```python
from build123d import *

# Parameters (mm, degrees)
BOSS_EXTRU_1_DEPTH      = 100
ESQUISSE3_R             = 2
ENL_V_MAT_EXTRU_2_DEPTH = 115.052675119
ESQUISSE7_W             = 5.5
ESQUISSE7_H             = 20.980762114
BOSS_EXTRU_3_DEPTH      = 29.226497
BOSS_EXTRU_4_OUTLINE_W  = 5.5
BOSS_EXTRU_4_OUTLINE_H  = 18.169872981
BOSS_EXTRU_4_DEPTH      = 10.490381057
CONG_2_R                = 40
CONG_3_R                = 40
CONG_4_R                = 5
CONG_5_RADIUS           = 5
CONG_5_LENGTH           = 100
ESQUISSE9_R             = 1.5
ENL_V_MAT_EXTRU_3_DEPTH = 112.741489915
CONG_6_R                = 1
CONG_7_R                = 1
CONG_8_R                = 30


# Read off the part's stored shape, not the designer's step: Boss.-Extru.4
with BuildPart() as part:
    # Esquisse1 → Boss.-Extru.1 (new body)
    with BuildSketch(Plane.XY):
        with BuildLine():
            Line((0, 0), (0, -24.226497308))
            ThreePointArc((0, -24.226497308), (1.339745962, -29.226497308), (5, -32.886751346))
            Line((5, -32.886751346), (30.310889132, -47.5))
            Line((30.310889132, -47.5), (35.310889132, -38.839745962))
            Line((35.310889132, -38.839745962), (10, -24.226497308))
            Line((10, -24.226497308), (10, 0))
            Line((10, 0), (0, 0))
        make_face()
    extrude(amount=BOSS_EXTRU_1_DEPTH)

    # Esquisse3 → Enlèv. mat.-Extru.2 (cut, through all)
    with BuildSketch(Plane(origin=(-7.990381057, -13.839745962, 0), x_dir=(0.86602540378444, -0.4999999999999978, 0), z_dir=(0.4999999999999978, 0.86602540378444, 0))):
        with Locations(Location((35.386751346, -50, 0), (0, 0, 180))):
            Circle(ESQUISSE3_R)
    extrude(amount=-ENL_V_MAT_EXTRU_2_DEPTH, mode=Mode.SUBTRACT)

    # Esquisse7 → Boss.-Extru.3 (add)
    with BuildSketch(Plane(origin=(43.301270189, -25, 0), x_dir=(0, 0, -1), z_dir=(0.86602540378444, -0.49999999999999756, 0))):
        with Locations((-97.25, -5.490381057)):
            Rectangle(ESQUISSE7_W, ESQUISSE7_H)
        with Locations((-2.75, -5.490381057)):
            Rectangle(ESQUISSE7_W, ESQUISSE7_H)
    extrude(amount=-BOSS_EXTRU_3_DEPTH)

    # Boss.-Extru.4 outline → Boss.-Extru.4 (add)
    with BuildSketch(Plane(origin=(10, 0, 0), x_dir=(0, 0, -1), z_dir=(1, 0, 0))):
        with Locations((-2.75, -15.141560818)):
            Rectangle(BOSS_EXTRU_4_OUTLINE_W, BOSS_EXTRU_4_OUTLINE_H)
        with Locations((-97.25, -15.141560818)):
            Rectangle(BOSS_EXTRU_4_OUTLINE_W, BOSS_EXTRU_4_OUTLINE_H)
    extrude(amount=BOSS_EXTRU_4_DEPTH)

    # Congé2
    # the kernel refuses this fillet: 40 mm, written as the material it takes off along each edge
    with BuildSketch(Plane(origin=(20.490381057, -6.056624327, 32.29491991), x_dir=(-1, 0, 0), z_dir=(0, 0, -1))) as cong_2_piece_1_section:
        with BuildLine():
            CenterArc((CONG_2_R * 0.267949192431, -CONG_2_R), CONG_2_R, 90, 30)
            Line((-CONG_2_R * 0.232050807569, -CONG_2_R * 0.133974596216), (0, 0))
            Line((0, 0), (CONG_2_R * 0.267949192431, 0))
        make_face()
    cong_2_piece_1 = extrude(amount=59.089839821, mode=Mode.PRIVATE)
    cong_2_piece_1 = split(cong_2_piece_1, bisect_by=Plane(origin=(10, -7.066001807, 2.75), z_dir=(1, 0, 0)), keep=Keep.TOP, mode=Mode.PRIVATE)
    add(cong_2_piece_1, mode=Mode.SUBTRACT)
    with BuildSketch(Plane(origin=(20.490381057, -6.056624327, 67.70508009), x_dir=(-1, 0, 0), z_dir=(0, 0, 1))) as cong_2_piece_2_section:
        with BuildLine():
            CenterArc((CONG_2_R * 0.267949192431, CONG_2_R), CONG_2_R, 240, 30)
            Line((-CONG_2_R * 0.232050807569, CONG_2_R * 0.133974596216), (0, 0))
            Line((0, 0), (CONG_2_R * 0.267949192431, 0))
        make_face()
    cong_2_piece_2 = extrude(amount=59.089839821, mode=Mode.PRIVATE)
    cong_2_piece_2 = split(cong_2_piece_2, bisect_by=Plane(origin=(10, -7.066001807, 97.25), z_dir=(1, 0, 0)), keep=Keep.TOP, mode=Mode.PRIVATE)
    add(cong_2_piece_2, mode=Mode.SUBTRACT)

    # Congé3
    # the kernel refuses this fillet: 40 mm, written as the material it takes off along each edge
    with BuildSketch(Plane(origin=(45.801270189, -20.669872981, -2.92475776), x_dir=(-0.8660254037844402, 0.49999999999999756, 0), z_dir=(0, 0, 1))) as cong_3_piece_1:
        with BuildLine():
            CenterArc((38.969903104, 40), CONG_3_R, 193.031161189, 76.968838811)
            Line((0, 30.980762114), (-0.779398062, 30.800377356))
            ThreePointArc((-0.779398062, 30.800377356), (-0.8, 15.490381057), (-0.8, 0))
            Line((-0.8, 0), (0, -0.8))
            Line((0, -0.8), (38.969903104, -0.8))
            Line((38.969903104, -0.8), (38.969903104, 0))
        make_face()
    extrude(amount=200.349515521, mode=Mode.SUBTRACT)

    # Congé4
    cong_4_edges = [part.edges().sort_by_distance(p)[0] for p in [
        (30.310889132, -47.5, 50),
    ]]
    fillet(cong_4_edges, radius=CONG_4_R)

    # Congé5: full round fillet: the end face becomes a half cylinder, R = half its width
    cong_5_face = Plane((5, 0, 50), x_dir=(0, 0, -1), z_dir=(0, 1, 0))  # on the end face: x along it, z out of the body
    cong_5_slab = cong_5_face.offset(-CONG_5_RADIUS / 2) * Box(CONG_5_LENGTH, 2 * CONG_5_RADIUS, CONG_5_RADIUS, mode=Mode.PRIVATE)  # the body's end, R deep
    cong_5_round = Plane((5, -5, 50), x_dir=(0, 1, 0), z_dir=(0, 0, -1)) * Cylinder(CONG_5_RADIUS, CONG_5_LENGTH, mode=Mode.PRIVATE)  # its axis R under the face
    add(cong_5_slab - cong_5_round, mode=Mode.SUBTRACT)

    # Esquisse9 → Enlèv. mat.-Extru.3 (cut, through all)
    with BuildSketch(Plane(origin=(10, 0, 0), x_dir=(0, 0, -1), z_dir=(1, 0, 0))):
        with Locations(Location((-74.5, -15.141560818, 0), (0, 0, 90))):
            Circle(ESQUISSE9_R)
        with Locations(Location((-25.5, -15.141560818, 0), (0, 0, 270))):
            Circle(ESQUISSE9_R)
    extrude(amount=-ENL_V_MAT_EXTRU_3_DEPTH, mode=Mode.SUBTRACT)

    # Congé6
    cong_6_edges = [part.edges().sort_by_distance(p)[0] for p in [
        (10, -6.057271778, 97.25),
    ]]
    fillet(cong_6_edges, radius=CONG_6_R)

    # Congé7
    cong_7_edges = [part.edges().sort_by_distance(p)[0] for p in [
        (10, -6.057271778, 2.75),
    ]]
    fillet(cong_7_edges, radius=CONG_7_R)

    # Congé8
    cong_8_edges = [part.edges().sort_by_distance(p)[0] for p in [
        (20.24714696, -7.452480042, 97.25),
        (20.24714696, -7.452480042, 2.75),
    ]]
    fillet(cong_8_edges, radius=CONG_8_R)


solid = part.part
```
Work out the finished part from the listing and answer in its coordinate system (mm). A direction names the side the tool comes from. Give positions to 0.01 mm unless a question says otherwise; leave off trailing zeros. Order: outer loops, then holes, each group sorted by start corner. A loop starts at its lowest first (then second) coordinate and runs counter-clockwise, first axis right, second up. Notation, with made-up numbers: M -6.75,79.5 L 38.25,79.5 A33 ccw 38.25,112.5 Z; hole C 36,36.5 d5. An arc over 180 degrees is marked long. Return JSON: item names as keys, results as strings.
1) For a pull along Y with two mould halves and no side action, classify faces 3 (the cylindrical face through (19.391, -35.341, 48.226)), 4 (the cylindrical face through (5.07, -14.946, 24.013)), 5 (the flat face through (10, -15, 60)), 6 (the cylindrical face through (1.3, -29.16, 49.3)) as +Y half, -Y half, draft (parallel to the pull), parting line (faces both ways), or undercut.
Resolved:
{"face 3": "undercut", "face 4": "undercut", "face 5": "draft", "face 6": "-Y half"}
2) A tool of negligible diameter and unlimited length cuts with its end or side. For faces 1 (the flat face through (16, -22, 0)), 2 (the flat face through (18.72, -29.26, 49.38)), from which of +Z, -Z, +X, -X, +Y, -Y can it reach the whole face along a straight path? Write none if from no direction.
Resolved:
{"face 1": "-Z, +X, -X, +Y, -Y", "face 2": "+X, +Y"}
3) Section C-C, the plane x = 4 is taken. Write down the section's boundary in (y, z), plus the area to 3 significant figures.
Resolved:
{"outline": "M -32.23,0 L -0.1,0 L -0.1,100 L -32.23,100 Z; hole C -15.14,25.5 d3; hole C -15.14,74.5 d3", "area": "3,200 mm^2"}
4) Section D-D, the plane y = -15 is taken. Give the number of separate pieces and of enclosed holes in the cut face, plus the area to 3 significant figures.
Resolved:
{"separate pieces": "3", "enclosed holes": "0", "area": "1,100 mm^2"}
5) Each of these flat-tipped pins is pushed along its axis until it touches: pin 1 (1 mm diameter, centred on x = 24, z = 84, fed in from -Y); pin 2 (10 mm diameter, centred on x = 26, z = 15, fed in from +Y); pin 3 (9.5 mm diameter, centred on y = -13.5, z = 66, fed in from +X). Where does it stop, or does it pass through?
Resolved:
{"pin 1": "y = -44.14", "pin 2": "y = -30.58", "pin 3": "x = 10"}
6) Section A-A, the plane z = 74.5 is taken. Write down the section's boundary in (x, y), plus the area to 3 significant figures.
Resolved:
{"outline": "M 0,-24.23 A10 ccw 5,-32.89 L 24.34,-44.05 A5 ccw 31.8,-40.28 A40 ccw 32.04,-36.95 L 10,-24.23 L 10,-16.64 L 0,-16.64 Z; M 0,-13.64 L 10,-13.64 L 10,-5 A5 ccw 0,-5 Z", "area": "518 mm^2"}
7) Straight lines are drawn through the part: line 1 along Z through (x, y) = (25, -17); line 2 along X through (y, z) = (-19.5, 52); line 3 along Z through (x, y) = (19, -39.5). For each, find the intervals that lie inside material, in ascending order. Write a range as [from, to].
Resolved:
{"line 1": "[0, 5.5], [94.5, 100]", "line 2": "[0, 10]", "line 3": "[0, 48.17], [51.83, 100]"}
8) Section B-B, the plane z = 59 is taken. Write down the section's boundary in (x, y).
Resolved:
{"outline": "M 0,-24.23 A10 ccw 5,-32.89 L 24.34,-44.05 A5 ccw 31.8,-40.28 A40 ccw 32.04,-36.95 L 10,-24.23 L 10,-5 A5 ccw 0,-5 Z"}
